Input: part model. Units: mm. Frame: model coordinates. Give positions to 0.01 mm unless a question says otherwise; leave off trailing zeros. Loops run counter-clockwise (first coordinate to the right, second up) from the corner with the lowest first, then second, coordinate; pieces in that order, holes last. Notation, with made-up numbers: (-15.5, 84.25) - (20.5, 84.25) arc R13 cw to (20.5, 94.25) - close; hole circle Ø9 at (-4.5, 61). An arc over 180 degrees is marked (long way). Answer as a JSON object with one key per item and string values.
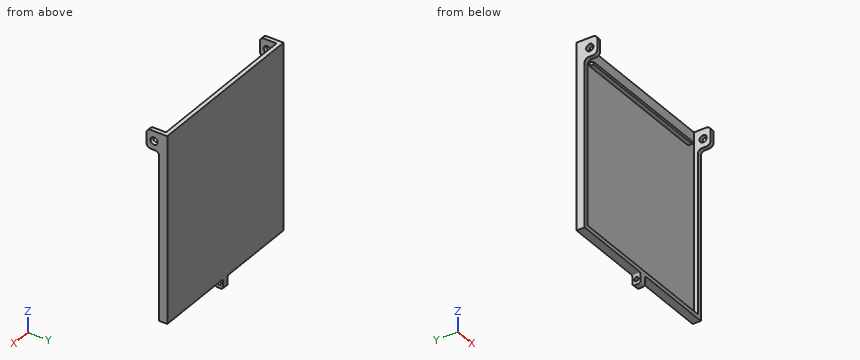
from build123d import *

# Parameters (mm, degrees)
BOSS_EXTRUDE2_DEPTH      = 8
SKETCH2_W                = 81
SKETCH2_H                = 89.6
BOSS_EXTRUDE3_DEPTH      = 2
SKETCH3_R                = 1.75
CUT_EXTRUDE1_DEPTH       = 125.5538661
CUT_EXTRUDE2_DEPTH       = 124.262587838
CUT_EXTRUDE2_DEPTH_BACK  = 124.262587838
SKETCH4_W                = 80.6
SKETCH4_H                = 6.1
SKETCH5_W                = 68.8
SKETCH5_H                = 1.2
BOSS_EXTRUDE4_DEPTH      = 2
FILLET2_R                = 2
BOSS_EXTRUDE5_DEPTH      = 1.5
BOSS_EXTRUDE5_DEPTH_BACK = 1.5
SKETCH7_R                = 1
FILLET5_R                = 1


with BuildPart() as part:
    # Sketch1 → Boss-Extrude2 (new body)
    with BuildSketch(Plane(origin=(0, 0, 0), x_dir=(1, 0, 0), z_dir=(0, 1, 0))):
        Polygon((-46.14154214, 4.488604838), (-46.14154214, 13.488604838), (-46.14154214, 92.088604838), (30.85845786, 92.088604838), (30.85845786, 13.488604838), (30.85845786, 4.488604838), (32.85845786, 4.488604838), (32.85845786, 94.088604838), (-48.14154214, 94.088604838), (-48.14154214, 4.488604838), align=None)
    extrude(amount=BOSS_EXTRUDE2_DEPTH)

    # Sketch2 → Boss-Extrude3 (add)
    with BuildSketch(Plane(origin=(0, 8, 0), x_dir=(1, 0, 0), z_dir=(0, 1, 0))):
        with Locations((-7.64154214, 49.288604838)):
            Rectangle(SKETCH2_W, SKETCH2_H)
    extrude(amount=BOSS_EXTRUDE3_DEPTH)

    # Sketch3 → Cut-Extrude1 (cut, through all)
    with BuildSketch(Plane(origin=(32.85845786, 0, 0), x_dir=(0, 0, -1), z_dir=(1, 0, 0))):
        with Locations((9.238604838, 3.6)):
            Circle(SKETCH3_R)
    extrude(amount=-CUT_EXTRUDE1_DEPTH, mode=Mode.SUBTRACT)

    # Sketch4 → Cut-Extrude2 (cut, two sides: drawn at the far end of the back side and taken through both)
    with BuildSketch(Plane.ZY.offset(-30.85845786).offset(-CUT_EXTRUDE2_DEPTH_BACK)):
        with Locations((-53.788604838, 3.05)):
            Rectangle(SKETCH4_W, SKETCH4_H)
    extrude(amount=CUT_EXTRUDE2_DEPTH + CUT_EXTRUDE2_DEPTH_BACK, mode=Mode.SUBTRACT)

    # Sketch5 → Boss-Extrude4 (add)
    with BuildSketch(Plane.XZ.offset(-8)):
        with Locations((-7.64154214, -12.405302831)):
            Rectangle(SKETCH5_W, SKETCH5_H)
    extrude(amount=BOSS_EXTRUDE4_DEPTH)

    # Fillet2
    fillet2_edges = [part.edges().sort_by_distance(p)[0] for p in [
        (-7.64154214, 8, -11.805302831),
        (-47.14154214, 0, -4.488604838),
        (-47.14154214, 0, -13.488604838),
        (-47.14154214, 6.1, -13.488604838),
        (31.85845786, 6.1, -13.488604838),
        (31.85845786, 0, -4.488604838),
        (31.85845786, 0, -13.488604838),
    ]]
    fillet(fillet2_edges, radius=FILLET2_R - 0.0001)  # a hair under: the kernel refuses the full size

    # Sketch7 → Boss-Extrude5 (add, two sides: drawn at the far end of the back side and taken through both)
    with BuildSketch(Plane.ZY.offset(7.64154214).offset(-BOSS_EXTRUDE5_DEPTH_BACK)):
        with BuildLine():
            Line((-94.088604838, 10), (-98.088604838, 10))
            ThreePointArc((-98.088604838, 10), (-98.79571162, 9.707106781), (-99.088604838, 9))
            Line((-99.088604838, 9), (-99.088604838, 7.1))
            ThreePointArc((-99.088604838, 7.1), (-98.79571162, 6.392893219), (-98.088604838, 6.1))
            Line((-98.088604838, 6.1), (-94.088604838, 6.1))
            Line((-94.088604838, 6.1), (-94.088604838, 10))
        make_face()
        with Locations((-96.588604838, 8.05)):
            Circle(SKETCH7_R, mode=Mode.SUBTRACT)
    extrude(amount=BOSS_EXTRUDE5_DEPTH + BOSS_EXTRUDE5_DEPTH_BACK)

    # Fillet5
    fillet5_edges = [part.edges().sort_by_distance(p)[0] for p in [
        (-6.14154214, 8.05, -94.088604838),
        (-9.14154214, 8.05, -94.088604838),
    ]]
    fillet(fillet5_edges, radius=FILLET5_R)


solid = part.part
Item 1: Material intervals for line 1 (Z direction, x = 16.5, y = 6.25); line 2 (X direction, y = 7, z = -75.5); line 3 (Y direction, x = -36.5, z = -27), sorted ascending. Write a range as [from, to].
Geometry check:
{"line 1": "z = [-94.09, -92.09], [-13.01, -11.79]", "line 2": "x = [-48.14, -46.14], [30.86, 32.86]", "line 3": "y = [8, 10]"}
Item 2: Contact query for flat-ended pins moving along their axis: P1, Ø0.6, axis at x = 32, y = 3, coming from the -Z side; P2, Ø1.2, axis at x = 17, y = 9, coming from the -Z side; P3, Ø1.5, axis at x = -12, z = -31, coming from the -Y side; P4, Ø5.5, axis at y = 3.6, z = -9.24, coming from the -X side. Output: stop coordinate, or through.
Geometry check:
{"P1": "stops at z = -13.49", "P2": "stops at z = -94.09", "P3": "stops at y = 8", "P4": "stops at x = -48.14"}
Item 3: Cut plane B-B (z = -46). Return loops of the section in (x, y).
Geometry check:
{"outline": "(-48.14, 6.1) - (-46.14, 6.1) - (-46.14, 8) - (30.86, 8) - (30.86, 6.1) - (32.86, 6.1) - (32.86, 10) - (-48.14, 10) - close"}
